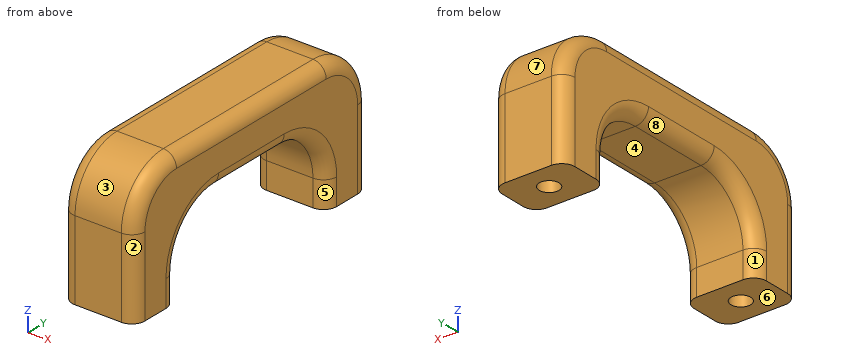
```python
from build123d import *

# Parameters (mm, degrees)
ESQUISSE1_W             = 11
ESQUISSE1_H             = 44.5
BOSS_EXTRU_1_DEPTH      = 20
CONG_1_R                = 8
ESQUISSE2_W             = 11.999855804
ESQUISSE2_H             = 28.501098838
ENL_V_MAT_EXTRU_1_DEPTH = 20
CONG_2_R                = 8
ESQUISSE3_R             = 1.5
ENL_V_MAT_EXTRU_2_DEPTH = 7
CONG_3_R                = 2


with BuildPart() as part:
    # Esquisse1 → Boss.-Extru.1 (new body)
    with BuildSketch(Plane.XY):
        Rectangle(ESQUISSE1_W, ESQUISSE1_H)
    extrude(amount=BOSS_EXTRU_1_DEPTH)

    # Congé1
    cong_1_edges = [part.edges().sort_by_distance(p)[0] for p in [
        (0, -22.25, 20),
        (0, 22.25, 20),
    ]]
    fillet(cong_1_edges, radius=CONG_1_R)

    # Esquisse2 → Enlèv. mat.-Extru.1 (cut)
    with BuildSketch(Plane(origin=(5.5, 0, 0), x_dir=(0, 0, -1), z_dir=(1, 0, 0))):
        with Locations((-5.999927902, 0)):
            Rectangle(ESQUISSE2_W, ESQUISSE2_H)
    extrude(amount=-ENL_V_MAT_EXTRU_1_DEPTH, mode=Mode.SUBTRACT)

    # Congé2
    cong_2_edges = [part.edges().sort_by_distance(p)[0] for p in [
        (0, -14.250549419, 11.999855804),
        (0, 14.250549419, 11.999855804),
    ]]
    fillet(cong_2_edges, radius=CONG_2_R)

    # Esquisse3 → Enlèv. mat.-Extru.2 (cut)
    with BuildSketch(Plane(origin=(0, 0, 0), x_dir=(-1, 0, 0), z_dir=(0, 0, -1))):
        with Locations((0, 18.25027471)):
            Circle(ESQUISSE3_R)
        with Locations((0, -18.25027471)):
            Circle(ESQUISSE3_R)
    extrude(amount=-ENL_V_MAT_EXTRU_2_DEPTH, mode=Mode.SUBTRACT)

    # Congé3
    cong_3_edges = [part.edges().sort_by_distance(p)[0] for p in [
        (5.5, 0, 20),
        (-5.5, 0, 20),
        (5.5, 22.25, 6),
        (5.5, -22.25, 6),
        (5.5, 19.906854249, 17.656854249),
        (5.5, -19.906854249, 17.656854249),
        (-5.5, -22.25, 6),
        (-5.5, 22.25, 6),
        (-5.5, 19.906854249, 17.656854249),
        (-5.5, -19.906854249, 17.656854249),
        (-5.5, 14.250549419, 1.999927902),
        (5.5, 14.250549419, 1.999927902),
        (5.5, -14.250549419, 1.999927902),
        (-5.5, -14.250549419, 1.999927902),
        (5.5, 0, 11.999855804),
        (-5.5, 0, 11.999855804),
        (5.5, -11.907403669, 9.656710053),
        (-5.5, -11.907403669, 9.656710053),
        (5.5, 11.907403669, 9.656710053),
        (-5.5, 11.907403669, 9.656710053),
    ]]
    fillet(cong_3_edges, radius=CONG_3_R)


solid = part.part
```
Check sheet for the modelled part. Datum: model origin and axes. Units: mm. Face numbers are marked on the shaded views. A direction names the side the tool comes from. Give positions to 0.01 mm unless a question says otherwise; leave off trailing zeros. Write each loop counter-clockwise with the first axis right and the second up, starting at its lowest first coordinate (ties: lowest second). Pieces come first, ordered by that corner, then holes. Notation, with made-up numbers: (89, 51) -> (131, 51) arc R21 cw to (131, 62) -> close; hole circle Ø7 at (4, 52). An arc over 180 degrees is marked (long way). Use CSV: the item, a comma, the result in double quotes. Start each with the question number.
Q1. Scan lines: line 1 along Y through (x, z) = (0, 4.25); line 2 along Y through (x, z) = (-3, 1.75); line 3 along Z through (x, y) = (-1, -4.5). Record each from-to range of solid material in increasing order.
Q2. Cross-section at B-B on x = 0. Enter the section's corners in (y, z), and give its area (3 significant figures).
Q3. Release check for a two-part mould opening along Y. For the marked faces 6, 7 and 8 record: +Y half, -Y half, draft (parallel to the pull), parting line (faces both ways), or undercut.
Q4. Depth check by flat-ended pin: P1, Ø0.9, axis at x = -0.5, y = 18, coming from the -Z side; P2, Ø5, axis at x = 4, z = 16.5, coming from the +Y side; P3, Ø2, axis at x = 1.5, y = -1.5, coming from the -Z side. Enter the tip coordinate at first touch or a pass-through.
Q5. Cross-section at A-A on y = -2. Enter the section's corners in (x, z), and give its area (3 significant figures).
Q6. Tool access check on the marked faces 1, 2, 3, 4 and 5. Record the directions out of +Z, -Z, +X, -X, +Y, -Y that give a thin tool (end or side, any length) a straight path to the whole face; none if there is none.
Working result:
1,line 1,"y = -22.25 to -19.75, -16.75 to -14.25, 14.25 to 16.75, 19.75 to 22.25"
1,line 2,"y = -22.25 to -14.25, 14.25 to 22.25"
1,line 3,"z = 12 to 20"
2,outline,"(-22.25, 0) -> (-19.75, 0) -> (-19.75, 7) -> (-16.75, 7) -> (-16.75, 0) -> (-14.25, 0) -> (-14.25, 4) arc R8 cw to (-6.25, 12) -> (6.25, 12) arc R8 cw to (14.25, 4) -> (14.25, 0) -> (16.75, 0) -> (16.75, 7) -> (19.75, 7) -> (19.75, 0) -> (22.25, 0) -> (22.25, 12) arc R8 ccw to (14.25, 20) -> (-14.25, 20) arc R8 ccw to (-22.25, 12) -> close"
2,area,"506 mm^2"
3,face 6,"draft"
3,face 7,"+Y half"
3,face 8,"undercut"
4,P1,"stops at z = 7"
4,P2,"stops at y = 21.99"
4,P3,"stops at z = 12"
5,outline,"(-5.5, 14) arc R2 ccw to (-3.5, 12) -> (3.5, 12) arc R2 ccw to (5.5, 14) -> (5.5, 18) arc R2 ccw to (3.5, 20) -> (-3.5, 20) arc R2 ccw to (-5.5, 18) -> close"
5,area,"84.6 mm^2"
6,face 1,"-Z, -X"
6,face 2,"+Z, -Z, +X, -Y"
6,face 3,"+Z, +X, -X, -Y"
6,face 4,"-Z, +X, -X"
6,face 5,"-Z, +X"
